The listing builds one solid part. Answer for the finished solid, in the listing's coordinates (mm). Coordinates: 2 decimals unless noted, no trailing zeros. Order: outer loops, then holes, each group sorted by start corner. A loop starts at its lowest first (then second) coordinate and runs counter-clockwise, first axis right, second up. Notation, with made-up numbers: (-27, 48) -> (10, 48) arc R13 ccw to (10, 64) -> close; hole circle Ø1 at (45, -8.75). An arc over 180 degrees is marked (long way). Put each result on its own line as item: value. Start each with the question number.
```python
from build123d import *

# Parameters (mm, degrees)
BOSS_EXTRUDE1_DEPTH      = 40
BOSS_EXTRUDE1_DEPTH_BACK = 40
SKETCH2_W                = 6.35
SKETCH2_H                = 12.7
SKETCH4_R                = 2.5
CUT_EXTRUDE1_DEPTH       = 41.995670503


with BuildPart() as part:
    # Sketch2 → Boss-Extrude1 (new, two sides: drawn at the far end of the back side and taken through both)
    with BuildSketch(Plane.XY.offset(-BOSS_EXTRUDE1_DEPTH_BACK)):
        Rectangle(SKETCH2_W, SKETCH2_H)
    extrude(amount=BOSS_EXTRUDE1_DEPTH + BOSS_EXTRUDE1_DEPTH_BACK)

    # Sketch4 → Cut-Extrude1 (cut, through all)
    with BuildSketch(Plane(origin=(3.175, 0, 0), x_dir=(0, 0, -1), z_dir=(1, 0, 0))):
        with Locations((-32, 0)):
            Circle(SKETCH4_R)
        with Locations(Location((32, 0, 0), (0, 0, 180))):
            Circle(SKETCH4_R)
    extrude(amount=-CUT_EXTRUDE1_DEPTH, mode=Mode.SUBTRACT)


solid = part.part
```
(1) The part is cut by section A-A on y = -1. Determine the outline of the cut face in (x, z) (3 decimals).
(2) The part is cut by section B-B on z = -32. Determine the outline of the cut face in (x, y) (3 decimals), plus the area to 3 significant figures.
(3) For a pull along Z with two mould halves and no side action, classify faces 1 (the cylindrical face through (0, -0.1, -34.5)), 2 (the flat face through (0, 0, -40)), 3 (the flat face through (0, -6.35, -1)) as released by +Z, released by -Z, zero draft, split by the parting line, or undercut.
(4) Find the intervals of material crossed by L1, parallel to Y at x = 1, z = 32; L2, parallel to Z at x = 0, y = -1; L3, parallel to Z at x = 1.75, y = 0.5, in increasing order.
(5) The part is cut by section C-C on x = -0.5. Determine the outline of the cut face in (y, z), plus the area to 3 significant figures.
Worked out:
1. outline: (-3.175, -40) -> (3.175, -40) -> (3.175, -34.291) -> (-3.175, -34.291) -> close; (-3.175, -29.709) -> (3.175, -29.709) -> (3.175, 29.709) -> (-3.175, 29.709) -> close; (-3.175, 34.291) -> (3.175, 34.291) -> (3.175, 40) -> (-3.175, 40) -> close
2. outline: (-3.175, -6.35) -> (3.175, -6.35) -> (3.175, -2.5) -> (-3.175, -2.5) -> close; (-3.175, 2.5) -> (3.175, 2.5) -> (3.175, 6.35) -> (-3.175, 6.35) -> close
2. area: 48.9 mm2
3. face 1: undercut
3. face 2: released by -Z
3. face 3: zero draft
4. L1: -6.35 to -2.5, 2.5 to 6.35
4. L2: -40 to -34.29, -29.71 to 29.71, 34.29 to 40
4. L3: -40 to -34.45, -29.55 to 29.55, 34.45 to 40
5. outline: (-6.35, -40) -> (6.35, -40) -> (6.35, 40) -> (-6.35, 40) -> close; hole circle Ø5 at (0, -32); hole circle Ø5 at (0, 32)
5. area: 977 mm2
